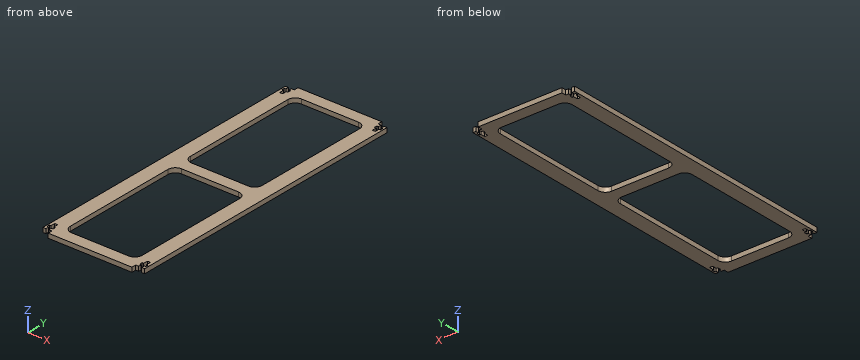
from build123d import *

# Parameters (mm, degrees)
SKETCH_1_W             = 68
SKETCH_1_H             = 200
EXTRUDE_1_DEPTH        = 3
SKETCH_2_W             = 6
SKETCH_2_H             = 3
CUT_EXTRUDE_1_DEPTH    = 212.265236137
SKETCH_3_W             = 48
SKETCH_3_H             = 88
CUT_EXTRUDE_2_DEPTH    = 212.265236137
FILLET_1_R             = 5
CUT_EXTRUDE_3_DEPTH    = 212.265236137
PATTERN_LINEAR_1_COUNT = 2
PATTERN_LINEAR_1_PITCH = 62
MIRROR_1_COPY_1_DEPTH  = 212.265236137


with BuildPart() as part:
    # 草图1 → 凸台-拉伸1 (new body)
    with BuildSketch(Plane.XY):
        with Locations((34, 100)):
            Rectangle(SKETCH_1_W, SKETCH_1_H)
    extrude(amount=EXTRUDE_1_DEPTH)

    # 草图2 → 切除-拉伸1 (cut, through all)
    with BuildSketch(Plane.XY.offset(3)):
        with Locations((65, 198.5)):
            Rectangle(SKETCH_2_W, SKETCH_2_H)
        with Locations((3, 198.5)):
            Rectangle(SKETCH_2_W, SKETCH_2_H)
        with Locations((65, 1.5)):
            Rectangle(SKETCH_2_W, SKETCH_2_H)
        with Locations((3, 1.5)):
            Rectangle(SKETCH_2_W, SKETCH_2_H)
    extrude(amount=-CUT_EXTRUDE_1_DEPTH, mode=Mode.SUBTRACT)

    # 草图3 → 切除-拉伸2 (cut, through all)
    with BuildSketch(Plane.XY.offset(3)):
        with Locations((34, 148)):
            Rectangle(SKETCH_3_W, SKETCH_3_H)
        with Locations((34, 52)):
            Rectangle(SKETCH_3_W, SKETCH_3_H)
    extrude(amount=-CUT_EXTRUDE_2_DEPTH, mode=Mode.SUBTRACT)

    # 圆角1
    fillet_1_edges = [part.edges().sort_by_distance(p)[0] for p in [
        (58, 192, 1.5),
        (58, 104, 1.5),
        (10, 104, 1.5),
        (10, 192, 1.5),
        (58, 96, 1.5),
        (58, 8, 1.5),
        (10, 8, 1.5),
        (10, 96, 1.5),
    ]]
    fillet(fillet_1_edges, radius=FILLET_1_R)

    # 草图4 → 切除-拉伸3 (cut, through all)
    with BuildSketch(Plane.XY.offset(3)):
        Polygon((2, 3), (4, 3), (4, 5), (5.05, 5), (5.05, 7), (4, 7), (4, 10), (2, 10), (2, 7), (0.95, 7), (0.95, 5), (2, 5), align=None)
    cut_extrude_3 = extrude(amount=-CUT_EXTRUDE_3_DEPTH, mode=Mode.SUBTRACT)

    # 阵列(线性)1: 切除-拉伸3 ×2
    with Locations(*[(i * PATTERN_LINEAR_1_PITCH, 0, 0) for i in range(1, PATTERN_LINEAR_1_COUNT)]):
        add(cut_extrude_3, mode=Mode.SUBTRACT)

    # 镜向1: 切除-拉伸3 across plane
    add(cut_extrude_3.mirror(Plane(origin=(0, 100, 0), x_dir=(0, 0, 1), z_dir=(0, -1, 0))), mode=Mode.SUBTRACT)

    # 镜向1 copy 1 sketch → 镜向1 copy 1 (cut, through all)
    with BuildSketch(Plane(origin=(62, 200, 3), x_dir=(1, 0, 0), z_dir=(0, 0, 1))):
        Polygon((2, -3), (4, -3), (4, -5), (5.05, -5), (5.05, -7), (4, -7), (4, -10), (2, -10), (2, -7), (0.95, -7), (0.95, -5), (2, -5), align=None)
    extrude(amount=-MIRROR_1_COPY_1_DEPTH, mode=Mode.SUBTRACT)


solid = part.part
For this review, take the finished solid that the model builds, in its own axes (mm). Round coordinates to 2 decimals unless told otherwise and drop trailing zeros. Order: outer loops, then holes, each group sorted by start corner. A loop starts at its lowest first (then second) coordinate and runs counter-clockwise, first axis right, second up. Notation, with made-up numbers: M 12.5,-14 L 46.5,-14 A21 ccw 46.5,-7 Z; hole C 87.25,-23 d6. An arc over 180 degrees is marked long. Use a Markdown table: item, result. Add a question column.
Item 1: Add section C-C, the plane z = 1.75. State how many separate pieces and enclosed holes the cut face has, then the cut area to 3 significant figures.
Item 2: Add section B-B, the plane y = 70. Give the boundary of the cut face in (x, z).
Item 3: To check wall thickness, follow line 1 along Y through (x, z) = (26, 0.9); line 2 along X through (y, z) = (25.5, 0.4); line 3 along X through (y, z) = (105.5, 0.75). State the ranges of each line that lie inside material, in increasing order.
Item 4: Add section A-A, the plane x = 56. Give the boundary of the cut face in (y, z).
Item 5: Add section D-D, the plane x = 37. Give the boundary of the cut face in (y, z), then the cut area to 3 significant figures.
Item 6: Insertion check: pin 1 (1.6 mm diameter, centred on x = 0.5, z = 1, fed in from -Y); pin 2 (1.5 mm diameter, centred on y = 2, z = 1.5, fed in from +X); pin 3 (1.2 mm diameter, centred on x = 1.5, z = 1, fed in from +Y). Each pin has a flat end and moves straight along its axis. Give the tip position at first contact, or say it passes through.
Geometry results:
| question | item | result |
|---|---|---|
| 1 | separate pieces | 1 |
| 1 | enclosed holes | 2 |
| 1 | area | 5,050 mm² |
| 2 | outline | M 0,0 L 10,0 L 10,3 L 0,3 Z; M 58,0 L 68,0 L 68,3 L 58,3 Z |
| 3 | line 1 | y = 0 to 8, 96 to 104, 192 to 200 |
| 3 | line 2 | x = 0 to 10, 58 to 68 |
| 3 | line 3 | x = 0 to 11.43, 56.57 to 68 |
| 4 | outline | M 0,0 L 9,0 L 9,3 L 0,3 Z; M 95,0 L 105,0 L 105,3 L 95,3 Z; M 191,0 L 200,0 L 200,3 L 191,3 Z |
| 5 | outline | M 0,0 L 8,0 L 8,3 L 0,3 Z; M 96,0 L 104,0 L 104,3 L 96,3 Z; M 192,0 L 200,0 L 200,3 L 192,3 Z |
| 5 | area | 72.0 mm² |
| 6 | pin 1 | stops at y = 3 |
| 6 | pin 2 | stops at x = 62 |
| 6 | pin 3 | stops at y = 197 |
